For this review, take the finished solid that the model builds, in its own axes (mm). A direction names the side the tool comes from. Coordinates: 2 decimals unless noted, no trailing zeros. Loops run counter-clockwise (first coordinate to the right, second up) from the corner with the lowest first, then second, coordinate; pieces in that order, holes last. Notation, with made-up numbers: (89.5, -13.75) - (127.5, -13.75) arc R20 cw to (127.5, -3.75) - close; hole circle Ø6 at (73.25, 66.5). An arc over 180 degrees is marked (long way). Use one line per item in the form item = value. Start each with the question number.
1. To check wall thickness, follow probe 1 along X at (y, z) = (-44, 0); probe 2 along Z at (x, y) = (0.5, -48) (3 decimals); probe 3 along Z at (x, y) = (-18.5, -50). State the ranges of each line that lie inside material, in increasing order.
2. Draft analysis for pull direction X (two halves, no side actions). For faces 1 (the face through (-24.397, -29.58, -12.69)), 2 (the face through (-22.3, -60, -12.1)), 3 (the face through (0, -10, 0)), state which applies: +X half, -X half, draft (parallel to the pull), parting line (faces both ways), or undercut.
3. Add section B-B on y = 71. Give the boundary of the cut face in (x, z), and give its area (3 significant figures).
4. Machinability: for faces 4 (the face through (7.509, -35.35, -23.846)), 5 (the face through (8.78, 59.16, 11.46)), which of the approach directions +Z, -Z, +X, -X, +Y, -Y give a long, thin tool a straight path to every point of the face, cutting with its end or side? Answer none if there is none.
5. For pin 1 Ø10 at (y, z) = (53.5, -16) entering from -X; pin 2 Ø10 at (x, z) = (13, -7) entering from -Y; pin 3 Ø3 at (y, z) = (33, -13.5) entering from +X, all flat-tipped, find the tip position at first contact; note any pin that passes through.
6. Add section A-A on y = -5. Give the boundary of the cut face in (x, z), and give its area (3 significant figures).
```python
from build123d import *

# Parameters (mm, degrees)
SKETCH3_R           = 27.5
BOSS_EXTRUDE1_DEPTH = 60
SKETCH4_R           = 25
CUT_EXTRUDE1_DEPTH  = 50


with BuildPart() as part:
    # Sketch2 → Revolve1 (revolve)
    with BuildSketch(Plane.XY, mode=Mode.PRIVATE) as revolve1_sk:
        Polygon((0, 0), (0, 120), (1, 120), (27.5, 0), align=None)
    revolve(revolve1_sk.sketch.rotate(Axis((0, 0, 0), (0, 1, 0)), 90), axis=Axis((0, 0, 0), (0, 1, 0)))

    # Sketch3 → Boss-Extrude1 (add)
    with BuildSketch(Plane.XZ):
        with Locations(Location((0, 0, 0), (0, 0, 270))):
            Circle(SKETCH3_R)
    extrude(amount=BOSS_EXTRUDE1_DEPTH)

    # Sketch4 → Cut-Extrude1 (cut)
    with BuildSketch(Plane.XZ.offset(60)):
        with Locations(Location((0, 0, 0), (0, 0, 270))):
            Circle(SKETCH4_R)
    extrude(amount=-CUT_EXTRUDE1_DEPTH, mode=Mode.SUBTRACT)


solid = part.part
```
Conclusion:
q1.probe_1 = -27.5 to -25, 25 to 27.5
q1.probe_2 = -27.495 to -24.995, 24.995 to 27.495
q1.probe_3 = -20.35 to -16.82, 16.82 to 20.35
q2.face_1 = parting line
q2.face_2 = draft
q2.face_3 = undercut
q3.outline = circle Ø23.64 at (0, 0)
q3.area = 439 mm^2
q4.face_4 = -Y
q4.face_5 = +Y
q5.pin_1 = -11.42
q5.pin_2 = -10
q5.pin_3 = 16.34
q6.outline = circle Ø55 at (0, 0)
q6.area = 2,380 mm^2
